```python
from build123d import *

# Parameters (mm, degrees)
BOSS_EXTRUDE1_DEPTH = 15
SKETCH3_R           = 7.5
BOSS_EXTRUDE2_DEPTH = 50
SKETCH4_R           = 20
SKETCH4_R_2         = 1.25
BOSS_EXTRUDE3_DEPTH = 5
SKETCH5_R           = 1.28
SKETCH5_W           = 20.5
SKETCH5_H           = 40.5
CUT_EXTRUDE1_DEPTH  = 10
SKETCH7_R           = 2.5
CUT_EXTRUDE2_DEPTH  = 10


with BuildPart() as part:
    # Sketch1 → Boss-Extrude1 (new body, symmetric)
    with BuildSketch(Plane.XY):
        Polygon((-52, 50), (-52, 0), (52, 0), (52, 50), (62, 50), (62, -10), (-62, -10), (-62, 50), align=None)
    extrude(amount=BOSS_EXTRUDE1_DEPTH, both=True)

    # Sketch3 → Boss-Extrude2 (add)
    with BuildSketch(Plane.XZ.offset(10)):
        Circle(SKETCH3_R)
    extrude(amount=BOSS_EXTRUDE2_DEPTH)

    # Sketch4 → Boss-Extrude3 (add)
    with BuildSketch(Plane.XZ.offset(60)):
        Circle(SKETCH4_R)
        with Locations((0, 15)):
            Circle(SKETCH4_R_2, mode=Mode.SUBTRACT)
        with Locations((-15, 0)):
            Circle(SKETCH4_R_2, mode=Mode.SUBTRACT)
        with Locations((15, 0)):
            Circle(SKETCH4_R_2, mode=Mode.SUBTRACT)
        with Locations((0, -15)):
            Circle(SKETCH4_R_2, mode=Mode.SUBTRACT)
    extrude(amount=BOSS_EXTRUDE3_DEPTH)

    # Sketch5 → Cut-Extrude1 (cut)
    with BuildSketch(Plane.ZY.offset(62)):
        with Locations((-4.8, 44.65)):
            Circle(SKETCH5_R)
        with Locations((5.2, 44.65)):
            Circle(SKETCH5_R)
        with Locations((-4.8, -4.537471889)):
            Circle(SKETCH5_R)
        with Locations((5.2, -4.537471889)):
            Circle(SKETCH5_R)
        with Locations((0, 20)):
            Rectangle(SKETCH5_W, SKETCH5_H)
    extrude(amount=-CUT_EXTRUDE1_DEPTH, mode=Mode.SUBTRACT)

    # Sketch7 → Cut-Extrude2 (cut)
    with BuildSketch(Plane(origin=(62, 0, 0), x_dir=(0, 0, -1), z_dir=(1, 0, 0))):
        with Locations((0, 30)):
            Circle(SKETCH7_R)
    extrude(amount=-CUT_EXTRUDE2_DEPTH, mode=Mode.SUBTRACT)


solid = part.part
```
Source: CAD feature listing. Evaluate the final solid. Frame: model axes, mm. A direction names the side the tool comes from. Give positions to 0.01 mm unless a question says otherwise; leave off trailing zeros. Order: outer loops, then holes, each group sorted by start corner. A loop starts at its lowest first (then second) coordinate and runs counter-clockwise, first axis right, second up.
(1) Pull-direction query (Y, two-part tool) for faces 5 (the face through (-57, -0.25, 0)), 6 (the face through (-7.493, -34.65, 0.33)), 7 (the face through (-57, 50, 0)), 8 (the face through (62, 20, 0)); classes: +Y half, -Y half, draft (parallel to the pull), parting line (faces both ways), or undercut.
(2) Access query for faces 1 (the face through (-4.336, -62.465, -19.524)), 2 (the face through (-57, 40.25, 0)), 3 (the face through (0, -60, -9)), 4 (the face through (52, 25, 0)). Directions: +Z, -Z, +X, -X, +Y, -Y. A direction counts if a zero-diameter tool reaches every point of the face in a straight line with its end or side. Return the directions, or none.
(3) Section query B-B (x = -40). Return the cut outline in (y, z).
(4) Contact query for flat-ended pins moving along their axis: P1, Ø0.8, axis at y = -4.5, z = 4.5, coming from the -X side; P2, Ø1.5, axis at x = -10.5, z = -1, coming from the +Y side; P3, Ø9, axis at y = 19, z = 3, coming from the -X side. Output: stop coordinate, or through.
(5) Section query C-C (y = -56). Return the cut outline in (x, z), plus the area to 3 significant figures.
(6) Section query A-A (y = 30). Return the cut outline in (x, z), plus the area to 3 significant figures.
(7) Material intervals for line 1 along Z through (x, y) = (0, -62.55); line 2 along X through (y, z) = (14, 13.5); line 3 along Y through (x, z) = (58, 0), sorted ascending.
Outcome:
1. face 5: undercut
1. face 6: undercut
1. face 7: +Y half
1. face 8: draft
2. face 1: -Y
2. face 2: -X
2. face 3: none
2. face 4: +Z, -Z, +Y
3. outline: (-10, -15) - (0, -15) - (0, 15) - (-10, 15) - close
4. P1: stops at x = -52
4. P2: stops at y = 0
4. P3: stops at x = 52
5. outline: circle Ø15 at (0, 0)
5. area: 177 mm2
6. outline: (-62, -15) - (-52, -15) - (-52, -10.25) - (-62, -10.25) - close; (-62, 10.25) - (-52, 10.25) - (-52, 15) - (-62, 15) - close; (52, -15) - (62, -15) - (62, -2.5) - (52, -2.5) - close; (52, 2.5) - (62, 2.5) - (62, 15) - (52, 15) - close
6. area: 345 mm2
7. line 1: z = -20 to -16.25, -13.75 to 13.75, 16.25 to 20
7. line 2: x = -62 to -52, 52 to 62
7. line 3: y = -10 to 27.5, 32.5 to 50
